from build123d import *

# Parameters (mm, degrees)
F0_R     = 60
F1_DEPTH = 40
F3_DEPTH = 100
F4_DEPTH = 25
F5_W     = 50
F5_H     = 20
F6_DEPTH = 15


with BuildPart() as f1:
    # F0 (on Top) → F1 (new body)
    with BuildSketch(Plane.XY):
        Circle(F0_R)
    extrude(amount=F1_DEPTH)

    # F2 (on Front) → F3 (cut, symmetric)
    with BuildSketch(Plane.XZ):
        with BuildLine():
            ThreePointArc((-60, 30.007477), (0.661156, 27.310043), (60, 14.427749))
            Line((60, 14.427749), (60, 41.473642))
            Line((60, 41.473642), (-60, 41.473642))
            Line((-60, 41.473642), (-60, 30.007477))
        make_face()
    extrude(amount=F3_DEPTH, both=True, mode=Mode.SUBTRACT)

    # F2 (on Front) → F4 (cut, symmetric)
    with BuildSketch(Plane.XZ):
        with BuildLine():
            ThreePointArc((-44.121098, 21.295034), (8.556291, 17.088967), (60, 5))
            Line((60, 5), (60, 14.427749))
            ThreePointArc((60, 14.427749), (0.661156, 27.310043), (-60, 30.007477))
            Line((-60, 30.007477), (-60, 27.070224))
            ThreePointArc((-60, 27.070224), (-52.563238, 22.800483), (-44.121098, 21.295034))
        make_face()
    extrude(amount=F4_DEPTH, both=True, mode=Mode.SUBTRACT)

    # F5 (on face) → F6 (cut)
    with BuildSketch(Plane(origin=(0, 0, 0), x_dir=(1, 0, 0), z_dir=(0, 0, -1))):
        with Locations((-33.5, 0)):
            Rectangle(F5_W, F5_H)
    extrude(amount=-F6_DEPTH, mode=Mode.SUBTRACT)


solid = f1.part
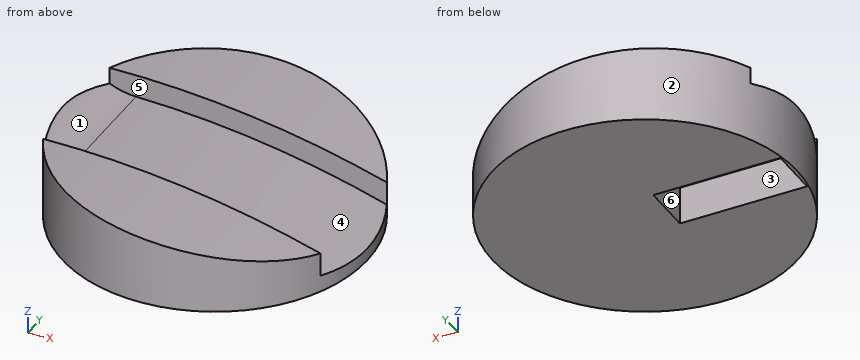
Source: CAD feature listing. Evaluate the final solid. Frame: model axes, mm. Face numbers are marked on the shaded views. A direction names the side the tool comes from. Round coordinates to 2 decimals unless told otherwise and drop trailing zeros. Loops run counter-clockwise (first coordinate to the right, second up) from the corner with the lowest first, then second, coordinate; pieces in that order, holes last. Notation, with made-up numbers: (-7, 23) - (40, 23) arc R25 cw to (40, 53) - close; hole circle Ø5 at (17.5, 25.5). An arc over 180 degrees is marked (long way). Write item = value, one per line. Start each with the question number.
Item 1: Section query D-D on x = -20. Output: boundary loops of the cut face in (y, z), plus the area to 3 significant figures.
Item 2: Reachability of the marked faces 1, 2 and 3 from +Z, -Z, +X, -X, +Y, -Y: full face, straight path, thin tool, end or side. Return the list, or none.
Item 3: Section query B-B on y = 0. Output: boundary loops of the cut face in (x, z).
Item 4: Material intervals for line 1 (Z direction, x = -42, y = 15.5); line 2 (Y direction, x = 31, z = 14); line 3 (Y direction, x = -31, z = 10), sorted ascending.
Item 5: First-contact query: pin 1 Ø3 at (y, z) = (24.5, 26) entering from -X; pin 2 Ø2 at (y, z) = (11, 10) entering from -X; pin 3 Ø1.5 at (y, z) = (33.5, 4) entering from +X. Flat tips, straight axial feed; report the tip coordinate or a pass-through.
Item 6: Mould query, pull axis X, two halves, no side actions, for the marked faces 4, 5 and 6. Classes: released by +X, released by -X, zero draft, split by the parting line, or undercut.
Item 7: Section query A-A on z = 2. Output: boundary loops of the cut face in (x, y).
Results list:
q1.outline = (-56.57, 0) - (-10, 0) - (-10, 15) - (10, 15) - (10, 0) - (56.57, 0) - (56.57, 29.39) - (25, 29.39) - (25, 20.36) - (-25, 20.36) - (-25, 29.39) - (-56.57, 29.39) - close
q1.area = 2,570 mm²
q2.face_1 = +Z, +X
q2.face_2 = +Z, -Z
q2.face_3 = -Z
q3.outline = (-60, 0) - (-58.5, 0) - (-58.5, 15) - (-8.5, 15) - (-8.5, 0) - (60, 0) - (60, 5) arc R350 ccw to (-44.12, 21.3) arc R25 cw to (-60, 27.07) - close
q4.line_1 = 0 to 21.28
q4.line_2 = -51.37 to -25, 25 to 51.37
q4.line_3 = -51.37 to -10, 10 to 51.37
q5.pin_1 = -54.54
q5.pin_2 = -59.16
q5.pin_3 = 50.27
q6.face_4 = released by +X
q6.face_5 = zero draft
q6.face_6 = undercut
q7.outline = circle Ø120 at (0, 0); hole (-58.5, -10) - (-8.5, -10) - (-8.5, 10) - (-58.5, 10) - close
